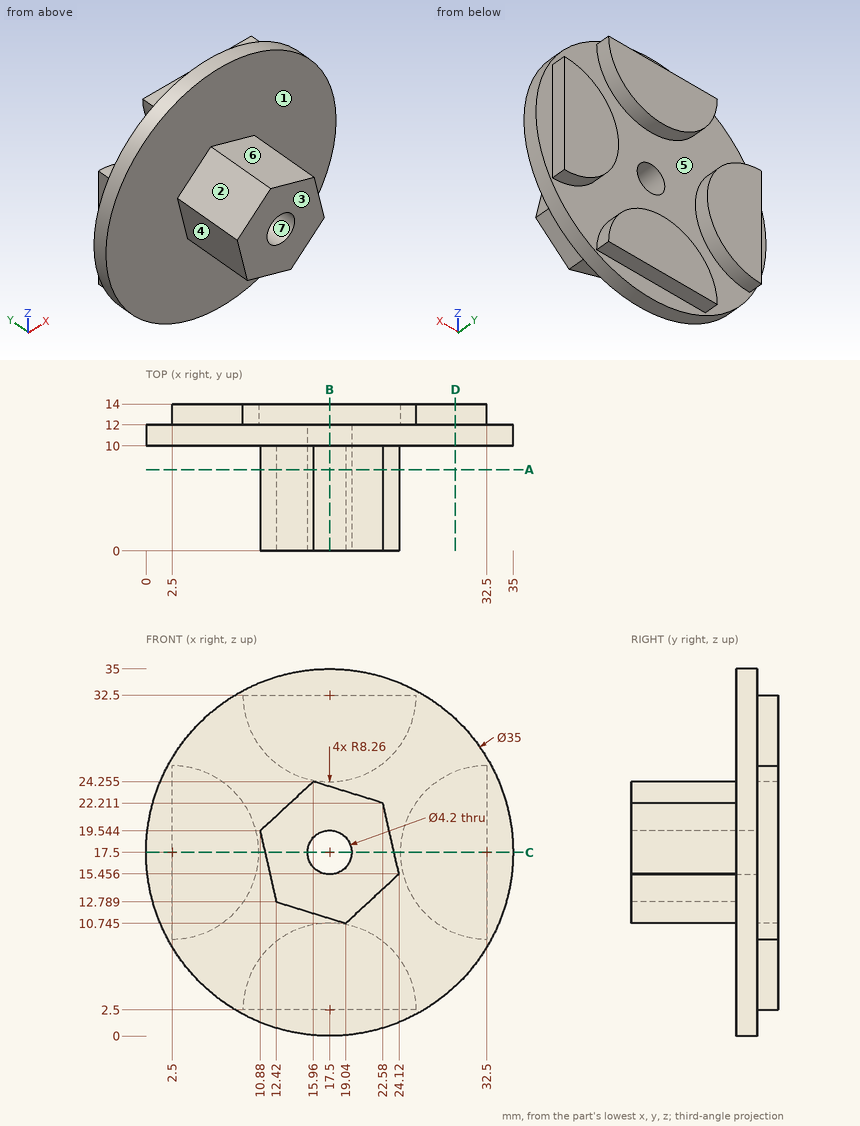
Verification items for this drawing (mm, ordinates from the low corner). A direction names the side the tool comes from. Give positions to 0.01 mm unless a question says otherwise; leave off trailing zeros. Loops run counter-clockwise (first coordinate to the right, second up) from the corner with the lowest first, then second, coordinate; pieces in that order, holes last. Notation, with made-up numbers: M -38.75,-31 L 6.25,-31 A17 cw 6.25,-8 Z; hole C -20.75,51.25 d9. An arc over 180 degrees is marked long. Return JSON: item names as keys, results as strings. Group by question number.
1. Cross-section at A-A on y = 7.75. Record the boundary of the cut face in (x, z) (1 decimal), plus the area to 3 significant figures.
2. Cross-section at C-C on z = 17.5. Record the boundary of the cut face in (x, y), plus the area to 3 significant figures.
3. Tool access check on the marked faces 1, 2 and 3. Record the directions out of +Z, -Z, +X, -X, +Y, -Y that give a thin tool (end or side, any length) a straight path to the whole face; none if there is none.
4. Cross-section at D-D on x = 29.5. Record the boundary of the cut face in (y, z).
5. Go/stop test with flat-tipped pins: pin 1 (1 mm diameter, centred on y = 10.5, z = 4, fed in from +X) (1 decimal); pin 2 (1 mm diameter, centred on x = 5, z = 10, fed in from -Y); pin 3 (1.5 mm diameter, centred on x = 16, y = 1.5, fed in from -Z); pin 4 (4 mm diameter, centred on x = 17.5, z = 17.5, fed in from +Y). Record where each tip stops, or that it passes through.
6. Cross-section at B-B on x = 17.5. Record the boundary of the cut face in (y, z), plus the area to 3 significant figures.
7. Thickness scan on L1, parallel to Y at x = 2.5, z = 26; L2, parallel to Y at x = 27, z = 11.5; L3, parallel to X at y = 8.25, z = 17.5 (1 decimal). Record the ranges inside material, lowest first.
8. Mould release check, pull along Z, two halves, no side actions. Record for the marked faces 4, 5, 6 and 7: released by +Z, released by -Z, zero draft, split by the parting line, or undercut.
Return value:
{
 "1": {"outline": "M 10.9,19.5 L 12.4,12.8 L 19,10.7 L 24.1,15.5 L 22.6,22.2 L 16,24.3 Z; hole C 17.5,17.5 d4.2", "area": "111 mm^2"},
 "2": {"outline": "M 0,10 L 11.35,10 L 11.35,0 L 15.4,0 L 15.4,12 L 10.76,12 L 10.76,14 L 2.5,14 L 2.5,12 L 0,12 Z; M 19.6,0 L 23.65,0 L 23.65,10 L 35,10 L 35,12 L 32.5,12 L 32.5,14 L 24.24,14 L 24.24,12 L 19.6,12 Z", "area": "176 mm^2"},
 "3": {"face 1": "-Y", "face 2": "+Z, -X, -Y", "face 3": "+Z, -Z, +X, -X, -Y"},
 "4": {"outline": "M 10,4.76 L 12,4.76 L 12,9.8 L 14,9.8 L 14,25.2 L 12,25.2 L 12,30.24 L 10,30.24 Z"},
 "5": {"pin 1": "x = 29.2", "pin 2": "y = 10", "pin 3": "z = 11.45", "pin 4": "through"},
 "6": {"outline": "M 0,11.22 L 10,11.22 L 10,0 L 12,0 L 12,2.5 L 14,2.5 L 14,10.76 L 12,10.76 L 12,15.4 L 0,15.4 Z; M 0,19.6 L 12,19.6 L 12,24.24 L 14,24.24 L 14,32.5 L 12,32.5 L 12,35 L 10,35 L 10,23.78 L 0,23.78 Z", "area": "178 mm^2"},
 "7": {"L1": "10 to 12", "L2": "10 to 14", "L3": "11.3 to 15.4, 19.6 to 23.7"},
 "8": {"face 4": "released by -Z", "face 5": "undercut", "face 6": "released by +Z", "face 7": "undercut"}
}
